Input: part model. Units: mm. Frame: model coordinates. Give positions to 0.01 mm unless a question says otherwise; leave off trailing zeros. Order: outer loops, then holes, each group sorted by start corner. A loop starts at its lowest first (then second) coordinate and runs counter-clockwise, first axis right, second up. Notation, with made-up numbers: M 46,11.5 L 97,11.5 A21 cw 97,18.5 Z; hole C 67.5,17.5 d4. An arc over 180 degrees is marked long. Use a Markdown table: item, result.
from build123d import *

# Parameters (mm, degrees)
F0_R     = 2.15265
F1_DEPTH = 3.175


with BuildPart() as f1:
    # F0 (on Top) → F1 (new body)
    with BuildSketch(Plane.XY):
        with BuildLine():
            ThreePointArc((355.6, 0), (177.8, 177.8), (0, 0))
            Line((0, 0), (0, -373.085176))
            ThreePointArc((0, -373.085176), (177.8, -550.885176), (355.6, -373.085176))
            Line((355.6, -373.085176), (355.6, 0))
        make_face()
        with Locations((105.56875, -445.316426)):
            Circle(F0_R, mode=Mode.SUBTRACT)
        with Locations((105.56875, -300.853926)):
            Circle(F0_R, mode=Mode.SUBTRACT)
        with Locations((250.03125, -445.316426)):
            Circle(F0_R, mode=Mode.SUBTRACT)
        with Locations((250.03125, -300.853926)):
            Circle(F0_R, mode=Mode.SUBTRACT)
        with Locations((250.03125, -261.9375)):
            Circle(F0_R, mode=Mode.SUBTRACT)
        with Locations((250.03125, -203.2)):
            Circle(F0_R, mode=Mode.SUBTRACT)
        with Locations((308.76875, -261.9375)):
            Circle(F0_R, mode=Mode.SUBTRACT)
        with Locations((308.76875, -203.2)):
            Circle(F0_R, mode=Mode.SUBTRACT)
        with Locations((114.497731, -184.255246)):
            Circle(F0_R, mode=Mode.SUBTRACT)
        with Locations((114.497731, 54.080246)):
            Circle(F0_R, mode=Mode.SUBTRACT)
        with Locations((241.102269, -184.255246)):
            Circle(F0_R, mode=Mode.SUBTRACT)
        with Locations((241.102269, 54.080246)):
            Circle(F0_R, mode=Mode.SUBTRACT)
        with Locations((177.8, 88.9)):
            Circle(F0_R, mode=Mode.SUBTRACT)
        with Locations((177.8, 165.1)):
            Circle(F0_R, mode=Mode.SUBTRACT)
    extrude(amount=F1_DEPTH)


solid = f1.part
1) Cut plane B-B on x = 82.5. Return loops of the section in (y, z) (3 decimals), and give its area (3 significant figures).
Response values:
| item | result |
|---|---|
| outline | M -523.188,0 L 150.102,0 L 150.102,3.175 L -523.188,3.175 Z |
| area | 2,140 mm² |
2) First-contact query: pin 1 Ø1 at (x, z) = (309, 2) entering from +Y. Flat tip, straight axial feed; report the tip coordinate or a pass-through.
Response values:
| item | result |
|---|---|
| pin 1 | stops at y = 120.54 |
3) Material intervals for line 1 (Y direction, x = 177.8, z = 1.05); line 2 (Y direction, x = 157, z = 2.6); line 3 (Y direction, x = 120.5, z = 0.8), sorted ascending. Write a range as from..to.
Response values:
| item | result |
|---|---|
| line 1 | y = -550.89..86.75, 91.05..162.95, 167.25..177.8 |
| line 2 | y = -549.66..176.58 |
| line 3 | y = -541.4..168.31 |
4) Cut plane C-C on x = 129.5. Return loops of the section in (y, z) (3 decimals).
Response values:
| item | result |
|---|---|
| outline | M -544.199,0 L 171.114,0 L 171.114,3.175 L -544.199,3.175 Z |
5) Cut plane A-A on z = 2.35. State how many separate pieces and enclosed holes the cut face has, and give its area (3 significant figures).
Response values:
| item | result |
|---|---|
| separate pieces | 1 |
| enclosed holes | 14 |
| area | 232,000 mm² |
